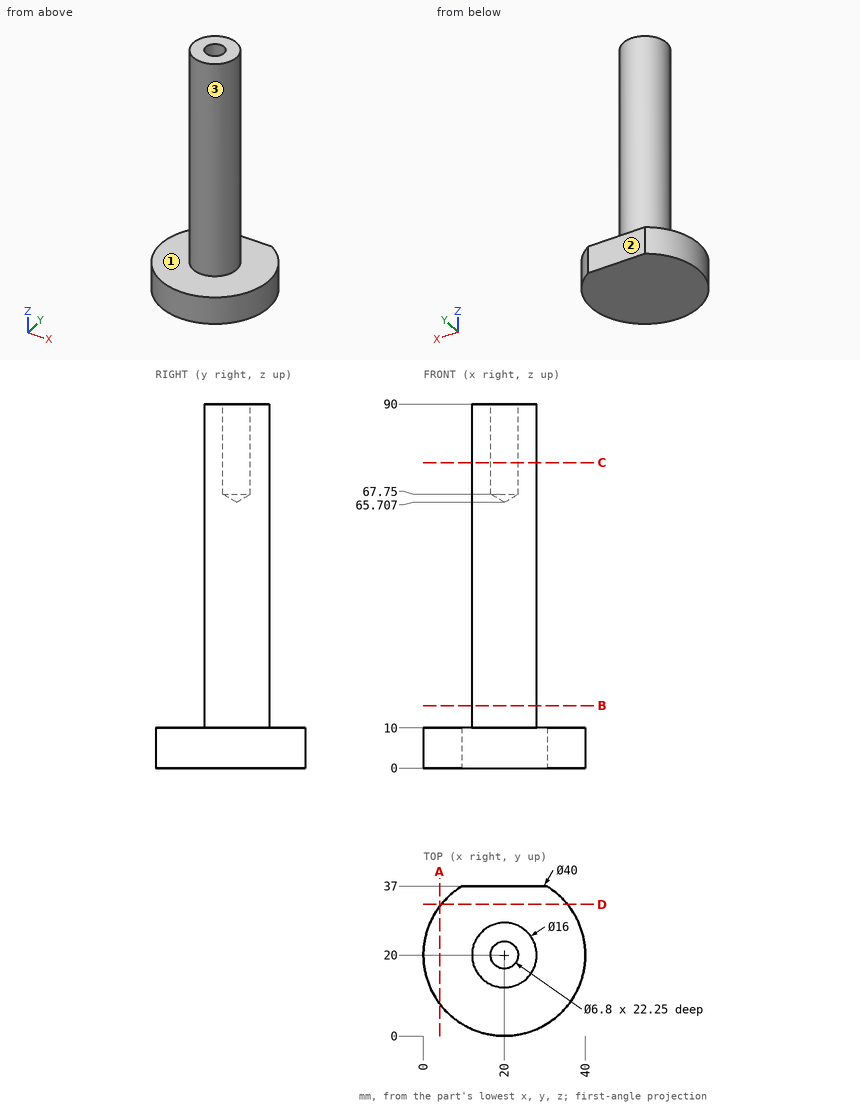
Part print with two shaded views. Sizes in mm from the minimum x, y, z corner. Give positions to 0.01 mm unless a question says otherwise; leave off trailing zeros. Loops run counter-clockwise (first coordinate to the right, second up) from the corner with the lowest first, then second, coordinate; pieces in that order, holes last. Notation, with made-up numbers: (-8.75, -38) -> (29.25, -38) arc R12 cw to (29.25, -27) -> close; hole circle Ø11 at (0, 46). An arc over 180 degrees is marked (long way). One line per question, with ' | ' between items.
Q1. Pull direction Y, two halves, no side cores. Call the marked faces 1, 2 and 3: pulls with the +Y half, pulls with the -Y half, needs draft (parallel to the pull), parting line crosses it, or undercut.
Filled sheet:
face 1: needs draft | face 2: pulls with the +Y half | face 3: parting line crosses it
Q2. Cut at D-D, the plane y = 32.5. Write the cut outline in (x, z), plus the area to 3 significant figures.
Filled sheet:
outline: (4.39, 0) -> (35.61, 0) -> (35.61, 10) -> (4.39, 10) -> close | area: 312 mm²
Q3. Cut at C-C, the plane z = 75.5. Write the cut outline in (x, y), plus the area to 3 significant figures.
Filled sheet:
outline: circle Ø16 at (20, 20); hole circle Ø6.8 at (20, 20) | area: 165 mm²
Q4. Cut at B-B, the plane z = 15.5. Write the cut outline in (x, y), plus the area to 3 significant figures.
Filled sheet:
outline: circle Ø16 at (20, 20) | area: 201 mm²
Q5. Cut at A-A, the plane x = 4. Write the cut outline in (y, z), plus the area to 3 significant figures.
Filled sheet:
outline: (8, 0) -> (32, 0) -> (32, 10) -> (8, 10) -> close | area: 240 mm²
Q6. Drill centre lines: line 1 along Y through (x, z) = (20, 77); line 2 along Z through (x, y) = (25, 33); line 3 along X through (y, z) = (22, 9). Where is each one in solid material? Low to high. Write a range as [from, to].
Filled sheet:
line 1: y = [12, 16.6], [23.4, 28] | line 2: z = [0, 10] | line 3: x = [0.1, 39.9]
Q7. Drop flat-ended pins along their axis: pin 1 (8 mm diameter, centred on x = 9, z = 75.5, fed in from +Y); pin 2 (12 mm diameter, centred on x = 30, z = 56.5, fed in from +Y); pin 3 (3 mm diameter, centred on x = 25.5, z = 37, fed in from -Y); pin 4 (12 mm diameter, centred on x = 34.5, z = 56.5, fed in from +Y) (1 decimal). Give the stop position or say it passes through.
Filled sheet:
pin 1: stops at y = 23.87 | pin 2: stops at y = 26.93 | pin 3: stops at y = 13.07 | pin 4: passes through
